Read the model definition and answer for the solid it produces. Units are mm, in the model's axes. A direction names the side the tool comes from. Give positions to 0.01 mm unless a question says otherwise; leave off trailing zeros. Order: outer loops, then holes, each group sorted by start corner. A loop starts at its lowest first (then second) coordinate and runs counter-clockwise, first axis right, second up. Notation, with made-up numbers: (49.25, 64.5) -> (105.25, 64.5) arc R20 ccw to (105.25, 81.5) -> close; hole circle Ø9 at (-37.5, 50.5). An arc over 180 degrees is marked (long way). One line per item, written item: value. Start each with the question number.
from build123d import *

# Parameters (mm, degrees)
SCHIZZO1_W                   = 30.00001
SCHIZZO1_H                   = 30.00001
ESTRUSIONE_ESTRUSIONE1_DEPTH = 58.2
TAGLIO_ESTRUSIONE1_REACH     = 74.023
SCHIZZO2_R                   = 6
TAGLIO_ESTRUSIONE2_REACH     = 74.023
SCHIZZO3_R                   = 6
SCHIZZO5_R                   = 7
TAGLIO_ESTRUSIONE3_DEPTH     = 20
FORO_6_0_6_1_D               = 6
FORO_FILETTATO_G1_8_1_D      = 8.8
FORO_FILETTATO_G1_8_1_DEPTH  = 10
FORO_FILETTATO_G1_8_1_TIP    = 2.643786724
FORO_FILETTATO_M3_1_REACH    = 74.023
FORO_FILETTATO_M3_1_BORE_R   = 1.25
FORO_4_0_4_2_D               = 4
FORO_4_0_4_2_DEPTH           = 8
FORO_4_0_4_2_TIP             = 1.201721238
TAGLIO_ESTRUSIONE5_DEPTH     = 10
TAGLIO_ESTRUSIONE6_START     = -10
TAGLIO_ESTRUSIONE6_DEPTH     = 10
SCHIZZO23_R                  = 1.6
TAGLIO_ESTRUSIONE7_DEPTH     = 10.00001
ESTRUSIONE_ESTRUSIONE2_START = 7
SCHIZZO24_R                  = 7
SCHIZZO24_R_2                = 3
ESTRUSIONE_ESTRUSIONE2_DEPTH = 7
FORO_FILETTATO_M3_2_D        = 2.5
FORO_FILETTATO_M3_2_DEPTH    = 11.5
FORO_FILETTATO_M3_2_TIP      = 0.751075774


with BuildPart() as part:
    # Schizzo1 → Estrusione-Estrusione1 (new body)
    with BuildSketch(Plane.XY):
        with Locations((15.000005, 15.000005)):
            Rectangle(SCHIZZO1_W, SCHIZZO1_H)
    extrude(amount=ESTRUSIONE_ESTRUSIONE1_DEPTH)

    # Schizzo2 → Taglio-Estrusione1 (cut, up to next)
    with BuildSketch(Plane.XZ, mode=Mode.PRIVATE) as taglio_estrusione1_sk1:
        with Locations(Location((22.00001, 50.2, 0), (0, 0, 270))):
            Circle(SCHIZZO2_R)
    taglio_estrusione1_tool1 = extrude(taglio_estrusione1_sk1.sketch, amount=-TAGLIO_ESTRUSIONE1_REACH, mode=Mode.PRIVATE) & part.part
    add(taglio_estrusione1_tool1.solids().sort_by_distance((22.00001, 0, 50.2))[0], mode=Mode.SUBTRACT)

    # Schizzo3 → Taglio-Estrusione2 (cut, up to next)
    with BuildSketch(Plane.ZY, mode=Mode.PRIVATE) as taglio_estrusione2_sk1:
        with Locations((16.6, 8)):
            Circle(SCHIZZO3_R)
    taglio_estrusione2_tool1 = extrude(taglio_estrusione2_sk1.sketch, amount=-TAGLIO_ESTRUSIONE2_REACH, mode=Mode.PRIVATE) & part.part
    add(taglio_estrusione2_tool1.solids().sort_by_distance((0, 8, 16.6))[0], mode=Mode.SUBTRACT)

    # Schizzo5 → Taglio-Estrusione3 (cut)
    with BuildSketch(Plane(origin=(0, 0, 0), x_dir=(-1, 0, 0), z_dir=(0, 0, -1))):
        with Locations((-9, 21.00001)):
            Circle(SCHIZZO5_R)
    extrude(amount=-TAGLIO_ESTRUSIONE3_DEPTH, mode=Mode.SUBTRACT)

    # Foro Ø6.0 (6)-1 (through all)
    with Locations(Plane.XY.offset(58.2)):
        with Locations((9, 21.00001)):
            Hole(FORO_6_0_6_1_D / 2)

    # Foro filettato G1/8-1
    with Locations(Plane(origin=(9, 21.00001, 58.2), x_dir=(1, 0, 0), z_dir=(0, 0, 1))):
        with Locations((0, 0)):
            Hole(FORO_FILETTATO_G1_8_1_D / 2, depth=FORO_FILETTATO_G1_8_1_DEPTH)
            with Locations((0, 0, -(FORO_FILETTATO_G1_8_1_DEPTH + FORO_FILETTATO_G1_8_1_TIP / 2))):  # 118° drill point
                Cone(0, FORO_FILETTATO_G1_8_1_D / 2, FORO_FILETTATO_G1_8_1_TIP, mode=Mode.SUBTRACT)

    # Foro filettato M3-1 bore → Foro filettato M3-1 (cut, up to next)
    with BuildSketch(Plane(origin=(30.00001, 0, 0), x_dir=(0, 0, -1), z_dir=(1, 0, 0)), mode=Mode.PRIVATE) as foro_filettato_m3_1_sk1:
        with Locations((-6, 21.00001)):
            Circle(FORO_FILETTATO_M3_1_BORE_R)
    foro_filettato_m3_1_tool1 = extrude(foro_filettato_m3_1_sk1.sketch, amount=-FORO_FILETTATO_M3_1_REACH, mode=Mode.PRIVATE) & part.part
    add(foro_filettato_m3_1_tool1.solids().sort_by_distance((30.00001, 21.00001, 6))[0], mode=Mode.SUBTRACT)

    # Foro Ø4.0 (4)-2
    with Locations(Plane(origin=(30.00001, 0, 0), x_dir=(0, 0, -1), z_dir=(1, 0, 0))):
        with Locations((-6, 21.00001)):
            Hole(FORO_4_0_4_2_D / 2, depth=FORO_4_0_4_2_DEPTH)
            with Locations((0, 0, -(FORO_4_0_4_2_DEPTH + FORO_4_0_4_2_TIP / 2))):  # 118° drill point
                Cone(0, FORO_4_0_4_2_D / 2, FORO_4_0_4_2_TIP, mode=Mode.SUBTRACT)

    # Schizzo20 → Taglio-Estrusione5 (cut)
    with BuildSketch(Plane.ZY):
        with BuildLine():
            Line((4, 8), (0, 8))
            Line((0, 8), (0, 0))
            Line((0, 0), (8, 0))
            Line((8, 0), (8, 4))
            ThreePointArc((8, 4), (6.828427125, 6.828427125), (4, 8))
        make_face()
    extrude(amount=-TAGLIO_ESTRUSIONE5_DEPTH, mode=Mode.SUBTRACT)

    # Schizzo21 → Taglio-Estrusione6 (cut)
    with BuildSketch(Plane(origin=(30.00001, 0, 0), x_dir=(0, 0, -1), z_dir=(1, 0, 0)).offset(TAGLIO_ESTRUSIONE6_START)):
        with BuildLine():
            Line((-8, 0), (-8, 4))
            ThreePointArc((-8, 4), (-6.828427125, 6.828427125), (-4, 8))
            Line((-4, 8), (0, 8))
            Line((0, 8), (0, 0))
            Line((0, 0), (-8, 0))
        make_face()
    extrude(amount=TAGLIO_ESTRUSIONE6_DEPTH, mode=Mode.SUBTRACT)

    # Schizzo23 → Taglio-Estrusione7 (cut)
    with BuildSketch(Plane.ZY.offset(-10)):
        with Locations((3.6, 3.6)):
            Circle(SCHIZZO23_R)
    extrude(amount=-TAGLIO_ESTRUSIONE7_DEPTH, mode=Mode.SUBTRACT)

    # Schizzo24 → Estrusione-Estrusione2 (add)
    with BuildSketch(Plane(origin=(0, 0, 20), x_dir=(-1, 0, 0), z_dir=(0, 0, -1)).offset(ESTRUSIONE_ESTRUSIONE2_START)):
        with Locations((-9, 21.00001)):
            Circle(SCHIZZO24_R)
        with Locations(Location((-9, 21.00001, 0), (0, 0, 180))):
            Circle(SCHIZZO24_R_2, mode=Mode.SUBTRACT)
    extrude(amount=-ESTRUSIONE_ESTRUSIONE2_DEPTH)

    # Foro filettato M3-2
    with Locations(Plane(origin=(30.00001, 28.00001, 39.1), x_dir=(0, 0, 1), z_dir=(1, 0, 0))):
        with Locations((0, 0), (-20, 0)):
            Hole(FORO_FILETTATO_M3_2_D / 2, depth=FORO_FILETTATO_M3_2_DEPTH)
            with Locations((0, 0, -(FORO_FILETTATO_M3_2_DEPTH + FORO_FILETTATO_M3_2_TIP / 2))):  # 118° drill point
                Cone(0, FORO_FILETTATO_M3_2_D / 2, FORO_FILETTATO_M3_2_TIP, mode=Mode.SUBTRACT)


solid = part.part
Item 1: Find section A-A on z = 16.6. Write down the section's boundary in (x, y).
Item 2: Find section D-D on y = 7. Write down the section's boundary in (x, z), then the cut area to 3 significant figures.
Item 3: Find section B-B on x = 9. Write down the section's boundary in (y, z), then the cut area to 3 significant figures.
Item 4: A tool of negligible diameter and unlimited length cuts with its end or side. For faces 1 (the cylindrical face through (24.17, 29.22, 39.37)), 2 (the cylindrical face through (4.803, 22.322, 53.13)), 3 (the cylindrical face through (2.323, 23.103, 6.409)), from which of +Z, -Z, +X, -X, +Y, -Y can it reach the whole face along a straight path? Write none if from no direction.
Item 5: Flat-ended cylindrical pins translate along their axes: pin 1 (1 mm diameter, centred on y = 25.5, z = 18, fed in from -X); pin 2 (4.5 mm diameter, centred on x = 5, z = 2, fed in from -Y); pin 3 (4.5 mm diameter, centred on x = 23, z = 2.5, fed in from -Y); pin 4 (11.5 mm diameter, centred on x = 9, y = 21, fed in from -Z). Find the tip coordinate at first contact, or state that the pin passes through.
Item 6: For a pull along Z with two mould halves and no side action, classify faces 4 (the flat face through (5, 2, 8)), 5 (the conical face through (17.879, 27.785, 19.072)), 6 (the flat face through (25, 8, 2)) as +Z half, -Z half, draft (parallel to the pull), parting line (faces both ways), or undercut.
Item 7: Find the intervals of material crossed by line 1 (Y direction, x = 9, z = 16.75); line 2 (X direction, y = 11, z = 50); line 3 (Y direction, x = 9, z = 34.25), in increasing order. Write a range as from..to.
Item 8: Find section C-C on y = 3. Write down the section's boundary in (x, z).
Checks:
1. outline: (0, 0) -> (30, 0) -> (30, 2) -> (0, 2) -> close; (0, 14) -> (30, 14) -> (30, 30) -> (0, 30) -> close; hole circle Ø6 at (9, 21)
2. outline: (0, 6.65) -> (10, 6.65) -> (10, 0) -> (20, 0) -> (20, 6.65) -> (30, 6.65) -> (30, 10.68) -> (0, 10.68) -> close; (0, 22.52) -> (30, 22.52) -> (30, 58.2) -> (0, 58.2) -> close; hole circle Ø12 at (22, 50.2)
2. area: 1,150 mm2
3. outline: (0, 8) -> (4, 8) arc R4 cw to (8, 4) -> (8, 0) -> (14, 0) -> (14, 13) -> (18, 13) -> (18, 47.36) -> (16.6, 48.2) -> (16.6, 58.2) -> (0, 58.2) -> close; (24, 13) -> (28, 13) -> (28, 0) -> (30, 0) -> (30, 58.2) -> (25.4, 58.2) -> (25.4, 48.2) -> (24, 47.36) -> close; hole circle Ø12 at (8, 16.6)
3. area: 1,090 mm2
4. face 1: +X
4. face 2: +Z
4. face 3: -Z
5. pin 1: x = 0
5. pin 2: y = 7.99
5. pin 3: y = 7.93
5. pin 4: z = 13
6. face 4: -Z half
6. face 5: undercut
6. face 6: draft
7. line 1: 0..2, 14..18, 24..30
7. line 2: 0..16, 28..30
7. line 3: 0..18, 24..30
8. outline: (0, 8) -> (10, 8) -> (10, 5.08) -> (20, 5.08) -> (20, 8) -> (30, 8) -> (30, 13.28) -> (0, 13.28) -> close; (0, 19.92) -> (30, 19.92) -> (30, 58.2) -> (0, 58.2) -> close; (10, 0) -> (20, 0) -> (20, 2.12) -> (10, 2.12) -> close; hole circle Ø12 at (22, 50.2)
